Check sheet for the modelled part. Datum: model origin and axes. Units: mm. A direction names the side the tool comes from. Coordinates: 2 decimals unless noted, no trailing zeros. Write each loop counter-clockwise with the first axis right and the second up, starting at its lowest first coordinate (ties: lowest second). Pieces come first, ordered by that corner, then holes. Notation, with made-up numbers: M -9,35 L -4,35 A24 ccw -4,58 Z; hole C 39.25,19 d6. An arc over 180 degrees is marked long. Answer as CSV lines item,"result". Start each with the question number.
1) Draft check along X on faces 1 (the cylindrical face through (-3.695, -8.465, 18.013)), 2 (the flat face through (0, 11, 2)), 3 (the flat face through (-3, -9, -31)), 4 (the cylindrical face through (-3.695, -8.465, -21.237)). Enter one of: +X half, -X half, draft (parallel to the pull), parting line (faces both ways), or undercut.
2) Go/stop test with flat-tipped pins: pin 1 Ø2.5 at (x, z) = (-3.5, -19.75) entering from +Y; pin 2 Ø2 at (x, y) = (-4, 10.5) entering from -Z; pin 3 Ø3 at (y, z) = (-5, -12.5) entering from +X; pin 4 Ø3.5 at (x, y) = (-3, 1) entering from +Z. Record where each tip stops, or that it passes through.
3) Section check C-C (z = -19.75). Record the cut outline in (x, y), and give its area (3 significant figures).
4) Access from +Z, -Z, +X, -X, +Y, -Y to the whole of each face (thin tool, end or side, straight path). Record for faces 5 (the flat face through (-4, 5, -16)), 6 (the flat face through (-3, -9, 23)), 7 (the flat face through (-3, 5, 16)).
5) Material ranges on L1, parallel to X at y = -8.6, z = 19.5; L2, parallel to Z at x = -3.5, y = -8.2; L3, parallel to Z at x = -2.5, y = -7.25, recorded low to high. Write a range as [from, to].
6) Section check B-B (y = 0). Record the cut outline in (x, z), and give its area (3 significant figures).
Autodesk Inventor part; units mm, degrees
ref_plane "YZ Plane" through (0, 0, 0) normal (1, 0, 0) x (0, 1, 0)
ref_plane "XZ Plane" through (0, 0, 0) normal (0, 1, 0) x (-1, 0, 0)
ref_plane "XY Plane" through (0, 0, 0) normal (0, 0, 1) x (1, 0, 0)
sketch "Sketch1" plane through (0, 0, 0) normal (1, 0, 0) x (0, 1, 0)
  circle A0 centre (0, 0) radius 11
  line L0 (0, 16) -> (-11, 16)
  line L1 (-11, 16) -> (-11, -16)
  line L2 (-11, -16) -> (11, -16)
  line L3 (11, -16) -> (11, 16)
  line L4 (11, 16) -> (0, 16)
  line L5 (-11, 16) -> (-11, 23)
  line L6 (-11, 23) -> (-6, 23)
  line L7 (-6, 23) -> (-6, 16)
  line L8 (-11, -16) -> (-11, -31)
  line L9 (-11, -31) -> (-6, -31)
  line L10 (-6, -31) -> (-6, -16)
  point P0 (11, 0)
  point P1 (-11, 0)
  dimension "d0" = 22
  dimension "d4" = 7
  dimension "d5" = 5
  dimension "d6" = 15
extrude "Extrusion1" add sketch "Sketch1" against normal blind 7 contours L3 L2 L1 A0 | A0 L1 L0 L4 L3 | L5 L6 L7 L0 | L2 L10 L9 L8
sketch "Sketch2" plane through (0, 11, 16) normal (0, 1, 0) x (1, 0, 0)
  line L0 (-7, 16) -> (-7, 32)
  line L1 (0, 16) -> (0, 0)
  line L2 (-7, 32) -> (0, 32)
  line L3 (0, 32) -> (0, 0)
  line L4 (0, 0) -> (-7, 0)
  line L5 (-7, 0) -> (-7, 32)
extrude "Extrusion2" add sketch "Sketch2" along normal blind 5
sketch "Sketch3" plane through (0, -6, 23) normal (0, 1, 0) x (1, 0, 0)
  line L0 (0, 7) -> (0, 0)
  line L1 (-7, 0) -> (-7, 7)
  line L2 (0, 0) -> (-7, 0)
  line L3 (0, 7) -> (-7, 7)
  circle A0 centre (-3.5, 3.5) radius 1.5
  line L4 (0, 54) -> (0, 39)
  line L5 (-7, 39) -> (-7, 54)
  line L6 (0, 54) -> (-7, 54)
  line L7 (0, 39) -> (-7, 39)
  line L8 (0, 46.5) -> (0, 39)
  line L9 (0, 23) -> (0, 54)
  line L10 (0, 46.5) -> (0, 54)
  line L11 (0, 54) -> (0, 50.25)
  line L12 (-7, 54) -> (-7, 23)
  circle A1 centre (-3.5, 42.75) radius 1.5
  circle A2 centre (-3.5, 50.25) radius 1.5
  dimension "d11" = 3
  dimension "d12" = 3
extrude "Extrusion3" cut sketch "Sketch3" against normal blind 5 contours A0
extrude "Extrusion4" cut sketch "Sketch3" against normal blind 5 contours A1
extrude "Extrusion5" cut sketch "Sketch3" against normal blind 5 contours A2
thread "Thread1"
thread "Thread2"
thread "Thread3"
properties part number "aguanta rolinera"
Results found:
1,face 1,"undercut"
1,face 2,"+X half"
1,face 3,"draft"
1,face 4,"undercut"
2,pin 1,"passes through"
2,pin 2,"stops at z = -16"
2,pin 3,"stops at x = 0"
2,pin 4,"stops at z = 16"
3,outline,"M -7,-11 L -5,-11 L -5,-6 L -7,-6 Z; M -2,-11 L 0,-11 L 0,-6 L -2,-6 Z"
3,area,"20.0 mm2"
4,face 5,"-Z, +X, -X, +Y"
4,face 6,"+Z, +X, -X, +Y, -Y"
4,face 7,"+Z, +X, -X, +Y"
5,L1,"x = [-7, -5], [-2, 0]"
5,L2,"z = [-31, -28.75], [-25.75, -21.25], [-18.25, -7.33], [7.33, 18], [21, 23]"
5,L3,"z = [-31, -28.37], [-26.13, -20.87], [-18.63, -8.27], [8.27, 18.38], [20.62, 23]"
6,outline,"M -7,-16 L 0,-16 L 0,-11 L -7,-11 Z; M -7,11 L 0,11 L 0,16 L -7,16 Z"
6,area,"70.0 mm2"
